Autodesk Fusion 360 part; units mm, degrees
sketch "Sketch1" plane through (0, 0, 0) normal (0, 0, 1) x (1, 0, 0)
  line L0 (0, 0) -> (61, 0)
  line L1 (61, 0) -> (61, 84)
  line L2 (61, 84) -> (0, 84)
  line L3 (0, 84) -> (0, 0)
  dimension "d1" = 61
  dimension "d2" = 84
extrude "Extrude1" add sketch "Sketch1" along normal blind 2
sketch "Sketch2" plane through (0, 0, 2) normal (0, 0, 1) x (-1, 0, 0)
  line L0 (0, -84) -> (0, 0)
  line L1 (0, 0) -> (-61, 0)
  line L2 (-61, 0) -> (-61, -84)
  line L3 (-61, -84) -> (0, -84)
  line L4 (-2, -2) -> (-59, -2)
  line L5 (-59, -2) -> (-59, -82)
  line L6 (-59, -82) -> (-2, -82)
  line L7 (-2, -82) -> (-2, -2)
  dimension "d5" = 57
  dimension "d6" = 80
extrude "Extrude2" add sketch "Sketch2" along normal blind 1 contours L4 L5 L6 L7
sketch "Sketch3" plane through (0, 0, 3) normal (0, 0, 1) x (-1, 0, 0)
  line L0 (-2, -82) -> (-2, -2)
  line L1 (-2, -2) -> (-59, -2)
  line L2 (-59, -2) -> (-59, -82)
  line L3 (-59, -82) -> (-2, -82)
  line L4 (-59, -82) -> (-53, -82)
  line L5 (-53, -82) -> (-53, -76)
  line L6 (-53, -76) -> (-59, -76)
  line L7 (-59, -76) -> (-59, -82)
extrude "Extrude3" cut sketch "Sketch3" against normal blind 1 contours L2 L3 L4 L5 L6 L7
sketch "Sketch4" plane through (0, 0, 3) normal (0, 0, 1) x (-1, 0, 0)
  line L0 (-53, -76) -> (-53, -82)
  line L1 (-53, -82) -> (-2, -82)
  line L2 (-2, -82) -> (-2, -2)
  line L3 (-2, -2) -> (-59, -2)
  line L4 (-59, -2) -> (-59, -76)
  line L5 (-59, -76) -> (-53, -76)
  line L6 (-2, -82) -> (-8, -82)
  line L7 (-8, -82) -> (-8, -76)
  line L8 (-8, -76) -> (-2, -76)
  line L9 (-2, -76) -> (-2, -82)
extrude "Extrude4" cut sketch "Sketch4" against normal blind 1 contours L1 L2 L6 L7 L8 L9
sketch "Sketch5" plane through (0, 0, 3) normal (0, 0, 1) x (-1, 0, 0)
  line L0 (-8, -76) -> (-2, -76)
  line L1 (-2, -76) -> (-2, -2)
  line L2 (-2, -2) -> (-59, -2)
  line L3 (-59, -2) -> (-59, -76)
  line L4 (-59, -76) -> (-53, -76)
  line L5 (-53, -76) -> (-53, -82)
  line L6 (-53, -82) -> (-8, -82)
  line L7 (-8, -82) -> (-8, -76)
  line L8 (-2, -2) -> (-8, -2)
  line L9 (-8, -2) -> (-8, -8)
  line L10 (-8, -8) -> (-2, -8)
  line L11 (-2, -8) -> (-2, -2)
extrude "Extrude5" cut sketch "Sketch5" against normal blind 1 contours L1 L2 L8 L9 L10 L11
sketch "Sketch6" plane through (0, 0, 2) normal (0, 0, 1) x (-1, 0, 0)
  line L0 (-8, -82) -> (-53, -82)
  line L1 (-53, -82) -> (-53, -76)
  line L2 (-53, -76) -> (-59, -76)
  line L3 (-59, -76) -> (-59, -2)
  line L4 (-59, -2) -> (-8, -2)
  line L5 (-8, -2) -> (-8, -8)
  line L6 (-8, -8) -> (-2, -8)
  line L7 (-2, -8) -> (-2, -76)
  line L8 (-2, -76) -> (-8, -76)
  line L9 (-8, -76) -> (-8, -82)
  line L10 (0, -84) -> (0, 0)
  line L11 (0, 0) -> (-61, 0)
  line L12 (-61, 0) -> (-61, -84)
  line L13 (-61, -84) -> (0, -84)
  line L14 (-14.5, 0) -> (-45.5, 0)
  line L15 (-45.5, 0) -> (-45.5, -2)
  line L16 (-45.5, -2) -> (-14.5, -2)
  line L17 (-14.5, -2) -> (-14.5, 0)
  dimension "d15" = 31
  dimension "d16" = 2
extrude "Extrude6" add sketch "Sketch6" along normal blind 1 contours L4 L11 L14 L15 L16 L17
sketch "Sketch7" plane through (0, 0, 3) normal (0, 0, 1) x (-1, 0, 0)
  line L0 (-8, -8) -> (-8, -2)
  line L1 (-8, -2) -> (-14.5, -2)
  line L2 (-14.5, -2) -> (-14.5, 0)
  line L3 (-14.5, 0) -> (-45.5, 0)
  line L4 (-45.5, 0) -> (-45.5, -2)
  line L5 (-45.5, -2) -> (-59, -2)
  line L6 (-59, -2) -> (-59, -76)
  line L7 (-59, -76) -> (-53, -76)
  line L8 (-53, -76) -> (-53, -82)
  line L9 (-53, -82) -> (-8, -82)
  line L10 (-8, -82) -> (-8, -76)
  line L11 (-8, -76) -> (-2, -76)
  line L12 (-2, -76) -> (-2, -8)
  line L13 (-2, -8) -> (-8, -8)
  line L14 (-53, -17) -> (-59, -17)
  line L15 (-59, -17) -> (-59, -22)
  line L16 (-59, -22) -> (-53, -22)
  line L17 (-53, -22) -> (-53, -17)
  dimension "d19" = 5
extrude "Extrude7" cut sketch "Sketch7" against normal blind 1 contours L6 L14 L15 L16 L17
sketch "Sketch8" plane through (0, 0, 3) normal (0, 0, 1) x (-1, 0, 0)
  line L0 (-53, -22) -> (-59, -22)
  line L1 (-59, -22) -> (-59, -76)
  line L2 (-59, -76) -> (-53, -76)
  line L3 (-53, -76) -> (-53, -82)
  line L4 (-53, -82) -> (-8, -82)
  line L5 (-8, -82) -> (-8, -76)
  line L6 (-8, -76) -> (-2, -76)
  line L7 (-2, -76) -> (-2, -8)
  line L8 (-2, -8) -> (-8, -8)
  line L9 (-8, -8) -> (-8, -2)
  line L10 (-8, -2) -> (-14.5, -2)
  line L11 (-14.5, -2) -> (-14.5, 0)
  line L12 (-14.5, 0) -> (-45.5, 0)
  line L13 (-45.5, 0) -> (-45.5, -2)
  line L14 (-45.5, -2) -> (-59, -2)
  line L15 (-59, -2) -> (-59, -17)
  line L16 (-59, -17) -> (-53, -17)
  line L17 (-53, -17) -> (-53, -22)
  line L18 (-5, -76) -> (-9, -76)
  line L19 (-9, -76) -> (-9, -46)
  line L20 (-9, -46) -> (-5, -46)
  line L21 (-5, -46) -> (-5, -76)
  dimension "d22" = 4
  dimension "d23" = 30
extrude "Extrude8" cut sketch "Sketch8" against normal blind 4 contours L6 L18 L19 L20 L21
sketch "Sketch9" plane through (0, 0, 2) normal (0, 0, 1) x (-1, 0, 0)
  line L0 (-45.5, -2) -> (-45.5, 0)
  line L1 (-45.5, 0) -> (-61, 0)
  line L2 (-61, 0) -> (-61, -84)
  line L3 (-61, -84) -> (0, -84)
  line L4 (0, -84) -> (0, 0)
  line L5 (0, 0) -> (-14.5, 0)
  line L6 (-14.5, 0) -> (-14.5, -2)
  line L7 (-14.5, -2) -> (-8, -2)
  line L8 (-8, -2) -> (-8, -8)
  line L9 (-8, -8) -> (-2, -8)
  line L10 (-2, -8) -> (-2, -76)
  line L11 (-2, -76) -> (-5, -76)
  line L12 (-5, -76) -> (-8, -76)
  line L13 (-8, -76) -> (-8, -82)
  line L14 (-8, -82) -> (-53, -82)
  line L15 (-53, -82) -> (-53, -76)
  line L16 (-53, -76) -> (-59, -76)
  line L17 (-59, -76) -> (-59, -22)
  line L18 (-59, -22) -> (-53, -22)
  line L19 (-53, -22) -> (-53, -17)
  line L20 (-53, -17) -> (-59, -17)
  line L21 (-59, -17) -> (-59, -2)
  line L22 (-59, -2) -> (-45.5, -2)
  circle A0 centre (-56, -79) radius 1.4
  dimension "d26" = 2.8
extrude "Extrude9" cut sketch "Sketch9" against normal blind 3.5 contours A0
sketch "Sketch10" plane through (0, 0, 2) normal (0, 0, 1) x (-1, 0, 0)
  circle A0 centre (-56, -79) radius 1.4
  line L0 (-45.5, -2) -> (-45.5, 0)
  line L1 (-45.5, 0) -> (-61, 0)
  line L2 (-61, 0) -> (-61, -84)
  line L3 (-61, -84) -> (0, -84)
  line L4 (0, -84) -> (0, 0)
  line L5 (0, 0) -> (-14.5, 0)
  line L6 (-14.5, 0) -> (-14.5, -2)
  line L7 (-14.5, -2) -> (-8, -2)
  line L8 (-8, -2) -> (-8, -8)
  line L9 (-8, -8) -> (-2, -8)
  line L10 (-2, -8) -> (-2, -76)
  line L11 (-2, -76) -> (-5, -76)
  line L12 (-5, -76) -> (-8, -76)
  line L13 (-8, -76) -> (-8, -82)
  line L14 (-8, -82) -> (-53, -82)
  line L15 (-53, -82) -> (-53, -76)
  line L16 (-53, -76) -> (-59, -76)
  line L17 (-59, -76) -> (-59, -22)
  line L18 (-59, -22) -> (-53, -22)
  line L19 (-53, -22) -> (-53, -17)
  line L20 (-53, -17) -> (-59, -17)
  line L21 (-59, -17) -> (-59, -2)
  line L22 (-59, -2) -> (-45.5, -2)
  circle A1 centre (-5, -79) radius 1.4
  dimension "d29" = 2.8
extrude "Extrude10" cut sketch "Sketch10" against normal blind 4.5 contours A1
sketch "Sketch11" plane through (0, 0, 2) normal (0, 0, 1) x (-1, 0, 0)
  circle A0 centre (-5, -79) radius 1.4
  circle A1 centre (-56, -79) radius 1.4
  line L0 (-45.5, -2) -> (-45.5, 0)
  line L1 (-45.5, 0) -> (-61, 0)
  line L2 (-61, 0) -> (-61, -84)
  line L3 (-61, -84) -> (0, -84)
  line L4 (0, -84) -> (0, 0)
  line L5 (0, 0) -> (-14.5, 0)
  line L6 (-14.5, 0) -> (-14.5, -2)
  line L7 (-14.5, -2) -> (-8, -2)
  line L8 (-8, -2) -> (-8, -8)
  line L9 (-8, -8) -> (-2, -8)
  line L10 (-2, -8) -> (-2, -76)
  line L11 (-2, -76) -> (-5, -76)
  line L12 (-5, -76) -> (-8, -76)
  line L13 (-8, -76) -> (-8, -82)
  line L14 (-8, -82) -> (-53, -82)
  line L15 (-53, -82) -> (-53, -76)
  line L16 (-53, -76) -> (-59, -76)
  line L17 (-59, -76) -> (-59, -22)
  line L18 (-59, -22) -> (-53, -22)
  line L19 (-53, -22) -> (-53, -17)
  line L20 (-53, -17) -> (-59, -17)
  line L21 (-59, -17) -> (-59, -2)
  line L22 (-59, -2) -> (-45.5, -2)
  circle A2 centre (-5, -5) radius 1.4
  dimension "d32" = 2.8
extrude "Extrude11" cut sketch "Sketch11" against normal blind 5 contours A2
sketch "Sketch12" plane through (0, 0, 2) normal (0, 0, 1) x (-1, 0, 0)
  circle A0 centre (-5, -5) radius 1.4
  circle A1 centre (-5, -79) radius 1.4
  circle A2 centre (-56, -79) radius 1.4
  line L0 (-45.5, -2) -> (-45.5, 0)
  line L1 (-45.5, 0) -> (-61, 0)
  line L2 (-61, 0) -> (-61, -84)
  line L3 (-61, -84) -> (0, -84)
  line L4 (0, -84) -> (0, 0)
  line L5 (0, 0) -> (-14.5, 0)
  line L6 (-14.5, 0) -> (-14.5, -2)
  line L7 (-14.5, -2) -> (-8, -2)
  line L8 (-8, -2) -> (-8, -8)
  line L9 (-8, -8) -> (-2, -8)
  line L10 (-2, -8) -> (-2, -76)
  line L11 (-2, -76) -> (-5, -76)
  line L12 (-5, -76) -> (-8, -76)
  line L13 (-8, -76) -> (-8, -82)
  line L14 (-8, -82) -> (-53, -82)
  line L15 (-53, -82) -> (-53, -76)
  line L16 (-53, -76) -> (-59, -76)
  line L17 (-59, -76) -> (-59, -22)
  line L18 (-59, -22) -> (-53, -22)
  line L19 (-53, -22) -> (-53, -17)
  line L20 (-53, -17) -> (-59, -17)
  line L21 (-59, -17) -> (-59, -2)
  line L22 (-59, -2) -> (-45.5, -2)
  circle A3 centre (-56, -19.5) radius 1.4
  dimension "d35" = 2.8
extrude "Extrude12" cut sketch "Sketch12" against normal blind 4.5 contours A3
The model under review builds one solid part; all positions refer to its coordinate system, in mm. A direction names the side the tool comes from. Round coordinates to 2 decimals unless told otherwise and drop trailing zeros. Loops run counter-clockwise (first coordinate to the right, second up) from the corner with the lowest first, then second, coordinate; pieces in that order, holes last. Notation, with made-up numbers: (-4.5, 2.25) -> (31.5, 2.25) arc R35 cw to (31.5, 41.25) -> close; hole circle Ø8 at (27, -9.5). An arc over 180 degrees is marked (long way). Answer as a JSON object with one key per item and string values. Group by question number.
1) For faces 5 (the face through (61, 41, 1)), 6 (the face through (7, 76, 1)), list the 3-axis set-ups (+Z, -Z, +X, -X, +Y, -Y) from which the entire face can be reached by the end or side of a thin tool; tool diameter is ignored.
2) We need section C-C on x = 56. Write out the cut boundary in (y, z), then the cut area to 3 significant figures.
3) Mouldability with a two-part tool opening along Y and no side actions: class faces 1 (the face through (9, 61, 2)), 2 (the face through (31, 84, 1)), 3 (the face through (30, 0, 1)), 4 (the face through (3.71, 5.54, 1.01)) as released by +Y, released by -Y, zero draft, split by the parting line, or undercut.
4) We need section D-D on y = 79. Write out the cut boundary in (x, z).
5) We need section A-A on z = 0.9. Write out the cut boundary in (x, y), then the cut area to 3 significant figures.
6) For pin 1 Ø3 at (x, y) = (56, 19.5) entering from +Z; pin 2 Ø0.5 at (x, z) = (10, 2.5) entering from -Y; pin 3 Ø0.5 at (x, z) = (6, 2.5) entering from -Y; pin 4 Ø2 at (x, y) = (5, 5) entering from -Z, all flat-tipped, find the tip position at first contact; note any pin that passes through.
7) For line 1 (X direction, y = 79, z = 1.3); line 2 (Y direction, x = 56, z = 1.5); line 3 (X direction, y = 69, z = 1.3), list the stretches that pass through material, from the lowest coordinate up. Write a range as [from, to].
8) We need section B-B on y = 19.5. Write out the cut boundary in (x, z), then the cut area to 3 significant figures.
Result set:
{
 "1": {"face 5": "+Z, -Z, +X, +Y, -Y", "face 6": "+Z, -Z"},
 "2": {"outline": "(0, 0) -> (18.1, 0) -> (18.1, 2) -> (17, 2) -> (17, 3) -> (2, 3) -> (2, 2) -> (0, 2) -> close; (20.9, 0) -> (77.6, 0) -> (77.6, 2) -> (76, 2) -> (76, 3) -> (22, 3) -> (22, 2) -> (20.9, 2) -> close; (80.4, 0) -> (84, 0) -> (84, 2) -> (80.4, 2) -> close", "area": "226 mm²"},
 "3": {"face 1": "undercut", "face 2": "released by +Y", "face 3": "released by -Y", "face 4": "undercut"},
 "4": {"outline": "(0, 0) -> (3.6, 0) -> (3.6, 2) -> (0, 2) -> close; (6.4, 0) -> (54.6, 0) -> (54.6, 2) -> (53, 2) -> (53, 3) -> (8, 3) -> (8, 2) -> (6.4, 2) -> close; (57.4, 0) -> (61, 0) -> (61, 2) -> (57.4, 2) -> close"},
 "5": {"outline": "(0, 0) -> (61, 0) -> (61, 84) -> (0, 84) -> close; hole circle Ø2.8 at (5, 5); hole circle Ø2.8 at (5, 79); hole (5, 46) -> (9, 46) -> (9, 76) -> (5, 76) -> close; hole circle Ø2.8 at (56, 19.5); hole circle Ø2.8 at (56, 79)", "area": "4,980 mm²"},
 "6": {"pin 1": "z = 2", "pin 2": "y = 2", "pin 3": "y = 8", "pin 4": "through"},
 "7": {"line 1": "[0, 3.6], [6.4, 54.6], [57.4, 61]", "line 2": "[0, 18.1], [20.9, 77.6], [80.4, 84]", "line 3": "[0, 5], [9, 61]"},
 "8": {"outline": "(0, 0) -> (54.6, 0) -> (54.6, 2) -> (53, 2) -> (53, 3) -> (2, 3) -> (2, 2) -> (0, 2) -> close; (57.4, 0) -> (61, 0) -> (61, 2) -> (57.4, 2) -> close", "area": "167 mm²"}
}
